Could you check a few things on this drawing? It's one solid part, dimensions in mm from its lowest x, y, z. Give positions to 0.01 mm unless a question says otherwise; leave off trailing zeros. Order: outer loops, then holes, each group sorted by start corner. A loop starts at its lowest first (then second) coordinate and runs counter-clockwise, first axis right, second up.
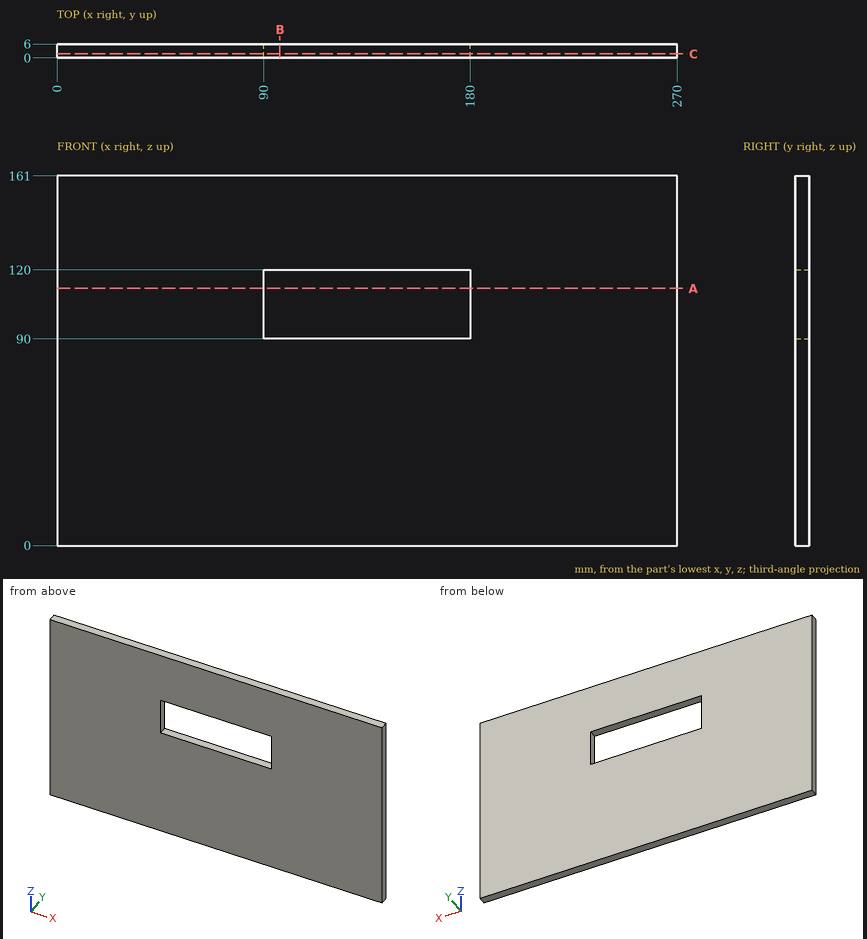
1) Suppose I cut it at C-C (y = 1.7). Please give me the cut outline in (x, z).
2) Suppose I cut it at A-A (z = 112). Please give me the cut outline in (x, y), and give its area (3 significant figures).
3) If I drill on line 1 (Z direction, x = 147.5, y = 4.15); line 2 (X direction, y = 3.65, z = 117), over which ranges is the centre line in solid material (lowest first)?
4) Suppose I cut it at B-B (x = 97). Please give me the cut outline in (y, z).
5) I'm going to push a flat-ended pin straight in: pin 1 Ø10 at (x, z) = (114, 55) entering from -Y. Where does the tip first touch, or does it pass through?
Results:
1. outline: (0, 0) - (270, 0) - (270, 161) - (0, 161) - close; hole (90, 90) - (180, 90) - (180, 120) - (90, 120) - close
2. outline: (0, 0) - (90, 0) - (90, 6) - (0, 6) - close; (180, 0) - (270, 0) - (270, 6) - (180, 6) - close
2. area: 1,080 mm2
3. line 1: z = 0 to 90, 120 to 161
3. line 2: x = 0 to 90, 180 to 270
4. outline: (0, 0) - (6, 0) - (6, 90) - (0, 90) - close; (0, 120) - (6, 120) - (6, 161) - (0, 161) - close
5. pin 1: stops at y = 0
